```python
from build123d import *

# Parameters (mm, degrees)
SKETCH1_R           = 0.8382
SKETCH1_R_2         = 2.159
BOSS_EXTRUDE1_DEPTH = 1.575
SKETCH2_W           = 86.242658642
SKETCH2_H           = 6.602
CUT_EXTRUDE1_DEPTH  = 65.362755899
CUT_EXTRUDE2_DEPTH  = 60.755092082
CUT_EXTRUDE3_DEPTH  = 60.755092082
SKETCH6_R           = 0.8382
CUT_EXTRUDE4_DEPTH  = 2.54


with BuildPart() as part:
    # Sketch1 → Boss-Extrude1 (new body)
    with BuildSketch(Plane(origin=(0, 0, 0), x_dir=(1, 0, 0), z_dir=(0, 1, 0))):
        Polygon((44.351293299, -40.014412246), (37.136293299, -40.014412246), (37.136293299, -46.615946892), (29.968293307, -46.615946892), (-30.083706693, -46.615946892), (-36.433706701, -46.615946892), (-36.433706701, -40.014412246), (-43.648706701, -40.014412246), (-43.648706701, -30.885946892), (-43.648706701, -29.647946892), (-42.378706693, -29.615946892), (-32.472706701, -29.647946892), (-32.472706701, -10.370428445), (-12.155556701, -10.370428445), (-12.155556701, -34.615947016), (-11.557706701, -34.615947016), (12.260293299, -34.615947016), (12.858143299, -34.615947016), (12.858143299, -10.370428445), (33.175293299, -10.370428445), (33.175293299, -12.929386892), (33.175293299, -29.647946892), (38.746293307, -29.615946892), (42.351293307, -29.615946892), (44.351293299, -29.647946892), (44.351293299, -31.651946892), align=None)
        with Locations(Location((-36.433706701, -35.965946892, 0), (0, 0, 270))):
            Circle(SKETCH1_R, mode=Mode.SUBTRACT)
        with Locations(Location((37.136293299, -35.983946892, 0), (0, 0, 270))):
            Circle(SKETCH1_R, mode=Mode.SUBTRACT)
        with Locations(Location((-19.648556701, -28.76738335, 0), (0, 0, 270))):
            Circle(SKETCH1_R_2, mode=Mode.SUBTRACT)
        with Locations(Location((-19.648556701, -20.63938335, 0), (0, 0, 270))):
            Circle(SKETCH1_R_2, mode=Mode.SUBTRACT)
        with Locations(Location((20.351397299, -20.63938335, 0), (0, 0, 270))):
            Circle(SKETCH1_R_2, mode=Mode.SUBTRACT)
        with Locations(Location((20.351397299, -28.76738335, 0), (0, 0, 270))):
            Circle(SKETCH1_R_2, mode=Mode.SUBTRACT)
        with Locations(Location((-25.868706701, -17.547875601, 0), (0, 0, 270))):
            Circle(SKETCH1_R, mode=Mode.SUBTRACT)
        with Locations(Location((26.571293299, -17.547875601, 0), (0, 0, 270))):
            Circle(SKETCH1_R, mode=Mode.SUBTRACT)
    extrude(amount=BOSS_EXTRUDE1_DEPTH)

    # Sketch2 → Cut-Extrude1 (cut, through all)
    with BuildSketch(Plane.XZ):
        with Locations((-5.985036022, 43.314946892)):
            Rectangle(SKETCH2_W, SKETCH2_H)
    extrude(amount=-CUT_EXTRUDE1_DEPTH, mode=Mode.SUBTRACT)

    # Sketch3 → Cut-Extrude2 (cut, through all)
    with BuildSketch(Plane.XZ):
        Polygon((-40.148706701, 40.013946892), (-40.148706701, 29.623150607), (-34.773706693, 29.640513821), (-34.773706693, 8.975624969), (-46.772834391, 8.975624969), (-46.772834391, 40.013946892), align=None)
    extrude(amount=-CUT_EXTRUDE2_DEPTH, mode=Mode.SUBTRACT)

    # Sketch4 → Cut-Extrude3 (cut, through all)
    with BuildSketch(Plane.XZ):
        Polygon((40.851293299, 40.014412246), (40.851293299, 32.420104455), (40.851293299, 29.615946892), (35.476293307, 29.615946892), (35.476293307, 10.370428445), (54.710892309, 10.370428445), (54.710892309, 40.014412246), align=None)
    extrude(amount=-CUT_EXTRUDE3_DEPTH, mode=Mode.SUBTRACT)

    # Sketch6 → Cut-Extrude4 (cut)
    with BuildSketch(Plane(origin=(0, 0, 0), x_dir=(-1, 0, 0), z_dir=(0, -1, 0))):
        with Locations(Location((27.141556701, -35.947946892, 0), (0, 0, 90))):
            Circle(SKETCH6_R)
        with Locations(Location((27.141556701, -25.025946892, 0), (0, 0, 90))):
            Circle(SKETCH6_R)
        with Locations(Location((14.695556701, -25.025946892, 0), (0, 0, 90))):
            Circle(SKETCH6_R)
        with Locations(Location((-15.398143299, -25.025946892, 0), (0, 0, 90))):
            Circle(SKETCH6_R)
        with Locations(Location((-27.844397299, -25.025946892, 0), (0, 0, 90))):
            Circle(SKETCH6_R)
        with Locations(Location((-27.844397299, -35.947946892, 0), (0, 0, 90))):
            Circle(SKETCH6_R)
    extrude(amount=-CUT_EXTRUDE4_DEPTH, mode=Mode.SUBTRACT)


solid = part.part
```
Verification items for the finished model (mm, model axes). A direction names the side the tool comes from. Coordinates: 2 decimals unless noted, no trailing zeros. Loops run counter-clockwise (first coordinate to the right, second up) from the corner with the lowest first, then second, coordinate; pieces in that order, holes last. Notation, with made-up numbers: (89.25, -29.5) - (147.25, -29.5) arc R22 ccw to (147.25, -5.5) - close; hole circle Ø1 at (54.25, 77.25). An arc over 180 degrees is marked (long way). Put each result on its own line as item: value.
Item 1: Draft check along Z on faces 4 (the face through (-12.156, 1, 22)), 5 (the face through (-2, 1, 40.014)), 6 (the face through (22.17, 0.78, 29.93)). Enter one of: pulls with the +Z half, pulls with the -Z half, needs draft (parallel to the pull), parting line crosses it, or undercut.
Conclusion:
face 4: needs draft
face 5: pulls with the +Z half
face 6: undercut
Item 2: Section check B-B (z = 25). Enter the section's corners in (x, y) (3 decimals).
Conclusion:
outline: (-32.473, 0) - (-27.979, 0) - (-27.979, 1.575) - (-32.473, 1.575) - close; (-26.304, 0) - (-15.533, 0) - (-15.533, 1.575) - (-26.304, 1.575) - close; (-13.858, 0) - (-12.156, 0) - (-12.156, 1.575) - (-13.858, 1.575) - close; (12.858, 0) - (14.56, 0) - (14.56, 1.575) - (12.858, 1.575) - close; (16.236, 0) - (27.007, 0) - (27.007, 1.575) - (16.236, 1.575) - close; (28.682, 0) - (33.175, 0) - (33.175, 1.575) - (28.682, 1.575) - close
Item 3: Section check C-C (z = 21). Enter the section's corners in (x, y) (3 decimals), then the cut area to 3 significant figures.
Conclusion:
outline: (-32.473, 0) - (-21.777, 0) - (-21.777, 1.575) - (-32.473, 1.575) - close; (-17.52, 0) - (-12.156, 0) - (-12.156, 1.575) - (-17.52, 1.575) - close; (12.858, 0) - (18.223, 0) - (18.223, 1.575) - (12.858, 1.575) - close; (22.48, 0) - (33.175, 0) - (33.175, 1.575) - (22.48, 1.575) - close
area: 50.6 mm2
Item 4: Section check A-A (z = 32.5). Enter the section's corners in (x, y) (3 decimals), then the cut area to 3 significant figures.
Conclusion:
outline: (-40.149, 0) - (-12.156, 0) - (-12.156, 1.575) - (-40.149, 1.575) - close; (12.858, 0) - (40.851, 0) - (40.851, 1.575) - (12.858, 1.575) - close
area: 88.2 mm2
Item 5: Scan lines: line 1 along X through (y, z) = (1.15, 20.5); line 2 along X through (y, z) = (0.4, 17.5); line 3 along X through (y, z) = (1.4, 12.75). Record each from-to range of solid material in increasing order.
Conclusion:
line 1: x = -32.47 to -21.8, -17.49 to -12.16, 12.86 to 18.2, 22.51 to 33.18
line 2: x = -32.47 to -26.71, -25.03 to -12.16, 12.86 to 25.73, 27.41 to 33.18
line 3: x = -32.47 to -12.16, 12.86 to 33.18
Item 6: Section check D-D (x = 7.5). Enter the section's corners in (y, z) (3 decimals), then the cut area to 3 significant figures.
Conclusion:
outline: (0, 34.616) - (1.575, 34.616) - (1.575, 40.014) - (0, 40.014) - close
area: 8.50 mm2
Item 7: Set-up check for faces 1 (the face through (23, 1, 10.37)), 2 (the face through (-32.473, 1, 20)), 3 (the face through (12.858, 1, 23)): record each of +Z, -Z, +X, -X, +Y, -Y from which the full face is reachable in a straight line by a thin tool's end or side.
Conclusion:
face 1: -Z, +X, -X, +Y, -Y
face 2: -Z, -X, +Y, -Y
face 3: -Z, +Y, -Y
